from build123d import *

# Parameters (mm, degrees)
SKETCH1_R           = 18
BOSS_EXTRUDE1_DEPTH = 89.8
SKETCH2_R           = 18.65
BOSS_EXTRUDE2_DEPTH = 18.65
BOSS_EXTRUDE4_DEPTH = 1.3
SKETCH3_R           = 18.65
BOSS_EXTRUDE3_DEPTH = 33.2
SKETCH11_R          = 4
CUT_EXTRUDE1_DEPTH  = 10.3
CUT_EXTRUDE2_DEPTH  = 6.7
SKETCH14_R          = 1.5
CUT_EXTRUDE3_DEPTH  = 10
SKETCH16_R          = 18.025
BOSS_EXTRUDE5_DEPTH = 20.5
SKETCH17_R          = 19.645678417
SKETCH17_R_2        = 17.75
CUT_EXTRUDE5_DEPTH  = 0.5
CUT_EXTRUDE6_DEPTH  = 3.5
SKETCH19_R          = 2.375
BOSS_EXTRUDE6_DEPTH = 3
CUT_EXTRUDE7_DEPTH  = 3


with BuildPart() as part:
    # Sketch1 → Boss-Extrude1 (new body)
    with BuildSketch(Plane(origin=(0, 0, 0), x_dir=(1, 0, 0), z_dir=(0, 1, 0))):
        Circle(SKETCH1_R)
    extrude(amount=BOSS_EXTRUDE1_DEPTH)

    # Sketch2 → Boss-Extrude2 (add)
    with BuildSketch(Plane(origin=(0, 89.8, 0), x_dir=(1, 0, 0), z_dir=(0, 1, 0))):
        Circle(SKETCH2_R)
    extrude(amount=BOSS_EXTRUDE2_DEPTH)

    # Sketch9 → Boss-Extrude4 (add)
    with BuildSketch(Plane.XZ):
        with BuildLine():
            Line((4.582575695, -10), (-4.582575695, -10))
            ThreePointArc((-4.582575695, -10), (-11, 0), (-4.582575695, 10))
            Line((-4.582575695, 10), (4.582575695, 10))
            ThreePointArc((4.582575695, 10), (11, 0), (4.582575695, -10))
        make_face()
    extrude(amount=BOSS_EXTRUDE4_DEPTH)

    # Sketch3 → Boss-Extrude3 (add)
    with BuildSketch(Plane(origin=(0, 69.8, 0), x_dir=(-1, 0, 0), z_dir=(0, -1, 0))):
        Circle(SKETCH3_R)
    extrude(amount=BOSS_EXTRUDE3_DEPTH)

    # Sketch11 → Cut-Extrude1 (cut)
    with BuildSketch(Plane.XZ.offset(1.3)):
        Circle(SKETCH11_R)
    extrude(amount=-CUT_EXTRUDE1_DEPTH, mode=Mode.SUBTRACT)

    # Sketch13 → Cut-Extrude2 (cut)
    with BuildSketch(Plane(origin=(0, 108.45, 0), x_dir=(1, 0, 0), z_dir=(0, 1, 0))):
        with BuildLine():
            Line((-16.522711642, -8.65), (16.522711642, -8.65))
            ThreePointArc((16.522711642, -8.65), (0, -18.65), (-16.522711642, -8.65))
        make_face()
    extrude(amount=-CUT_EXTRUDE2_DEPTH, mode=Mode.SUBTRACT)

    # Sketch14 → Cut-Extrude3 (cut)
    with BuildSketch(Plane.XZ):
        with Locations((-9.899494937, 9.899494937)):
            Circle(SKETCH14_R)
        with Locations((9.899494937, 9.899494937)):
            Circle(SKETCH14_R)
        with Locations((9.899494937, -9.899494937)):
            Circle(SKETCH14_R)
        with Locations((-9.899494937, -9.899494937)):
            Circle(SKETCH14_R)
    extrude(amount=-CUT_EXTRUDE3_DEPTH, mode=Mode.SUBTRACT)

    # Sketch16 → Boss-Extrude5 (add)
    with BuildSketch(Plane(origin=(0, 6.5, 0), x_dir=(-1, 0, 0), z_dir=(0, -1, 0))):
        Circle(SKETCH16_R)
    extrude(amount=-BOSS_EXTRUDE5_DEPTH)

    # Sketch17 → Cut-Extrude5 (cut)
    with BuildSketch(Plane(origin=(0, 31.5, 0), x_dir=(-1, 0, 0), z_dir=(0, -1, 0))):
        Circle(SKETCH17_R)
        Circle(SKETCH17_R_2, mode=Mode.SUBTRACT)
    extrude(amount=-CUT_EXTRUDE5_DEPTH, mode=Mode.SUBTRACT)

    # Sketch18 → Cut-Extrude6 (cut)
    with BuildSketch(Plane.XZ):
        with BuildLine():
            Line((2.75, -15), (2.75, -20))
            Line((2.75, -20), (-2.75, -20))
            Line((-2.75, -20), (-2.75, -15))
            ThreePointArc((-2.75, -15), (0, -12.25), (2.75, -15))
        make_face()
        with BuildLine():
            Line((2.75, 15), (2.75, 20))
            Line((2.75, 20), (-2.75, 20))
            Line((-2.75, 20), (-2.75, 15))
            ThreePointArc((-2.75, 15), (0, 12.25), (2.75, 15))
        make_face()
        with BuildLine():
            Line((-15, 2.75), (-20, 2.75))
            Line((-20, 2.75), (-20, -2.75))
            Line((-20, -2.75), (-15, -2.75))
            ThreePointArc((-15, -2.75), (-12.25, 0), (-15, 2.75))
        make_face()
        with BuildLine():
            Line((15, -2.75), (20, -2.75))
            Line((20, -2.75), (20, 2.75))
            Line((20, 2.75), (15, 2.75))
            ThreePointArc((15, 2.75), (12.25, 0), (15, -2.75))
        make_face()
    extrude(amount=-CUT_EXTRUDE6_DEPTH, mode=Mode.SUBTRACT)

    # Sketch19 → Boss-Extrude6 (add)
    with BuildSketch(Plane.XZ.offset(-3.5)):
        with Locations((-15, 0)):
            Circle(SKETCH19_R)
        with Locations((0, 15)):
            Circle(SKETCH19_R)
        with Locations((15, 0)):
            Circle(SKETCH19_R)
        with Locations((0, -15)):
            Circle(SKETCH19_R)
    extrude(amount=BOSS_EXTRUDE6_DEPTH)

    # Sketch20 → Cut-Extrude7 (cut)
    with BuildSketch(Plane.XZ.offset(-0.5)):
        Polygon((16.515813069, 0.875155083), (15, 1.750310167), (13.484186931, 0.875155083), (13.484186931, -0.875155083), (15, -1.750310167), (16.515813069, -0.875155083), align=None)
        Polygon((-1.750310167, 15), (-0.875155083, 13.484186931), (0.875155083, 13.484186931), (1.750310167, 15), (0.875155083, 16.515813069), (-0.875155083, 16.515813069), align=None)
        Polygon((0.875155083, -16.515813069), (1.750310167, -15), (0.875155083, -13.484186931), (-0.875155083, -13.484186931), (-1.750310167, -15), (-0.875155083, -16.515813069), align=None)
        Polygon((-16.515813069, -0.875155083), (-15, -1.750310167), (-13.484186931, -0.875155083), (-13.484186931, 0.875155083), (-15, 1.750310167), (-16.515813069, 0.875155083), align=None)
    extrude(amount=-CUT_EXTRUDE7_DEPTH, mode=Mode.SUBTRACT)


solid = part.part
The listing builds one solid part. Answer for the finished solid, in the listing's coordinates (mm). A direction names the side the tool comes from. Coordinates: 2 decimals unless noted, no trailing zeros. Order: outer loops, then holes, each group sorted by start corner. A loop starts at its lowest first (then second) coordinate and runs counter-clockwise, first axis right, second up.
Q1. For a pull along X with two mould halves and no side action, classify faces 6 (the face through (14.8, 53.43, 11.35)), 7 (the face through (8.4, 3.2, 9.97)), 8 (the face through (0, 105, 8.65)) as pulls with the +X half, pulls with the -X half, needs draft (parallel to the pull), parting line crosses it, or undercut.
Q2. A cutting plane is placed at A-A, the plane y = 65. Write down the section's boundary in (x, z).
Q3. Consider line 1 (Z direction, x = 0, y = 3) (3 decimals); line 2 (Y direction, x = 17, z = -5.5); line 3 (Y direction, x = -11, z = 4). Determine where each line is inside the solid, lowest interval first.
Q4. Given P1, Ø1, axis at x = 12.5, y = 43, coming from the +Z side; P2, Ø1, axis at y = 30.5, z = 10, coming from the +X side; P3, Ø1, axis at x = 1.5, y = 52.5, coming from the -Z side, each flat-ended and moving along its own axis, determine where each tip first touches the part or whether it passes through.
Q5. Which of the six approach directions +Z, -Z, +X, -X, +Y, -Y give full straight-line access (tool end or side, diameter ignored) to faces 1 (the face through (-2.75, 2, 16)), 2 (the face through (-9.8, 89.8, -15.3)), 3 (the face through (-11, -1, 0)), 4 (the face through (16, 2, -2.75)), 5 (the face through (12.25, 1.73, 0.06))?
Q6. A cutting plane is placed at B-B, the plane y = 80. Write down the section's boundary in (x, z).
Answers follow:
1. face 6: parting line crosses it
1. face 7: undercut
1. face 8: needs draft
2. outline: circle Ø37.3 at (0, 0)
3. line 1: z = -17.375 to -16.516, -13.484 to -12.625, -12.25 to -4, 4 to 12.25, 12.625 to 13.484, 16.516 to 17.375
3. line 2: y = 0 to 31.5, 32 to 108.45
3. line 3: y = 0 to 108.45
4. P1: stops at z = 14.28
4. P2: stops at x = 15.29
4. P3: stops at z = -18.62
5. face 1: +Z, -Y
5. face 2: none
5. face 3: -X, -Y
5. face 4: +X, -Y
5. face 5: -Y
6. outline: circle Ø36 at (0, 0)
